Check sheet for the modelled part. Datum: model origin and axes. Units: mm. A direction names the side the tool comes from. Give positions to 0.01 mm unless a question says otherwise; leave off trailing zeros. Write each loop counter-clockwise with the first axis right and the second up, starting at its lowest first coordinate (ties: lowest second). Pieces come first, ordered by that corner, then holes. Notation, with made-up numbers: M 1.25,-13.75 L 42.25,-13.75 A27 ccw 42.25,5.25 Z; hole C 37.25,-22.5 d3. An arc over 180 degrees is marked long. Write item = value, one per line. Start each with the question number.
1) Go/stop test with a flat-tipped pin: pin 1 (12.5 mm diameter, centred on x = -1, z = 11.5, fed in from -Y). Record where the tip stops, or that it passes through.
2) Mould release check, pull along Y, two halves, no side actions. Record for faces 3 (the flat face through (-25.171, 7.087, 12.325)), 4 (the cylindrical face through (35.1, -3.2, 9.4)), 5 (the flat face through (25, -7, 12)): released by +Y, released by -Y, zero draft, split by the parting line, or undercut.
3) Cross-section at B-B, the plane y = -5. Give the number of separate pieces and of enclosed holes in the cut face, plus the area to 3 significant figures.
4) Scan lines: line 1 along Z through (x, y) = (37.75, -3.1); line 2 along X through (y, z) = (-7.75, 22.5); line 3 along Z through (x, y) = (38.5, -5). Record each from-to range of solid material in increasing order. Write a range as [from, to].
5) Access from +Z, -Z, +X, -X, +Y, -Y to the whole of each face (thin tool, end or side, straight path). Record for faces 1 (the flat face through (-1, 3, 0)), 2 (the flat face through (-25, -7, 12)).
6) Cross-section at D-D, the plane x = 30. Record the cut outline in (y, z).
7) Cross-section at A-A, the plane z = 4.5. Record the cut outline in (x, y).
8) Cross-section at C-C, the plane x = -28. Record the cut outline in (y, z), plus the area to 3 significant figures.
Autodesk Inventor part; units mm, degrees
ref_plane "YZ Plane" through (0, 0, 0) normal (1, 0, 0) x (0, 1, 0)
ref_plane "XZ Plane" through (0, 0, 0) normal (0, 1, 0) x (-1, 0, 0)
ref_plane "XY Plane" through (0, 0, 0) normal (0, 0, 1) x (1, 0, 0)
sketch "Skizze1" plane through (0, 0, 0) normal (0, 0, 1) x (1, 0, 0)
  line L0 (-63, 0) -> (63, 0)
  line L1 (0, -6) -> (0, 18.5)
  arc A0 (5.8901, 13.979) -> (-5.8901, 13.979) centre (0, -2.5) ccw
  line L2 (-5.8901, 13.979) -> (-45, 0)
  line L3 (5.8901, 13.979) -> (45, 0)
  line L4 (-45, 0) -> (45, 0)
  dimension "d2" = 35
  dimension "d3" = 15
  dimension "d4" = 45
extrude "Extrusion1" add sketch "Skizze1" along normal blind 25
sketch "Skizze4" plane through (-45, 0, 0) normal (0, -1, 0) x (1, 0, 0)
  line L0 (0, 25) -> (90, 25)
  line L1 (0, 0) -> (0, 25)
  line L2 (90, 25) -> (0, 25)
  line L3 (0, 25) -> (0, 0)
  line L4 (0, 0) -> (90, 0)
  line L5 (90, 0) -> (90, 25)
  point P0 (45, 0)
extrude "Extrusion4" add sketch "Skizze4" along normal blind 10
sketch "Skizze5" plane through (-45, -10, 0) normal (-1, 0, 0) x (0, 0, 1)
  line L0 (25, 0) -> (0, 0)
  line L1 (0, 10) -> (0, 0)
  point P0 (4.5, 5)
  point P1 (20.5, 5)
  dimension "d17" = 5
  dimension "d18" = 5
  dimension "d19" = 25
  dimension "d20" = 16
  dimension "d21" = 4.5
hole "Bohrung1" at (-45, -5, 4.5) at (-45, -5, 20.5) direction (1, 0, 0) diameter 6 end through all
sketch "Skizze6" plane through (-45, -10, 0) normal (-1, 0, 0) x (0, 0, 1)
  line L0 (0, 10) -> (25, 10)
  line L1 (0, 23.979) -> (0, 10)
  point P0 (12.5, 6.9)
  dimension "d29" = 3.1
  dimension "d30" = 12.5
hole "Bohrung2" at (-45, -3.1, 12.5) direction (1, 0, 0) diameter 6.2 end through all
sketch "Skizze7" plane through (0, 0, 0) normal (0, 0, -1) x (-1, 0, 0)
  line L0 (0, -15) -> (0, 20)
  line L1 (45, -10) -> (-45, -10)
  line L2 (-25, -10) -> (25, -10)
  line L3 (25, -10) -> (25, 1)
  line L4 (25, 1) -> (-25, 1)
  line L5 (-25, 1) -> (-25, -10)
  point P0 (0, 0)
  dimension "d38" = 50
  dimension "d39" = 11
extrude "Extrusion5" cut sketch "Skizze7" against normal blind 25
properties part number "Schieber"
Reply:
q1.pin_1 = 1
q2.face_3 = released by +Y
q2.face_4 = undercut
q2.face_5 = zero draft
q3.separate_pieces = 8
q3.enclosed_holes = 0
q3.area = 324 mm2
q4.line_1 = [0, 2.18], [6.82, 9.4], [15.6, 18.18], [22.82, 25]
q4.line_2 = [-45, -25], [25, 45]
q4.line_3 = [0, 1.5], [7.5, 10.05], [14.95, 17.5], [23.5, 25]
q5.face_1 = -Z, +X, -X, +Y, -Y
q5.face_2 = +Z, -Z, -Y
q6.outline = M -10,0 L 5.36,0 L 5.36,25 L -10,25 Z; hole C -5,4.5 d6; hole C -5,20.5 d6; hole C -3.1,12.5 d6.2
q7.outline = M -45,-10 L -25,-10 L -25,-8 L -45,-8 Z; M -45,-2 L -25,-2 L -25,1 L 25,1 L 25,-2 L 45,-2 L 45,0 L 5.89,13.98 A17.5 ccw -5.89,13.98 L -45,0 Z; M 25,-10 L 45,-10 L 45,-8 L 25,-8 Z
q8.outline = M -10,0 L 6.08,0 L 6.08,25 L -10,25 Z; hole C -5,4.5 d6; hole C -5,20.5 d6; hole C -3.1,12.5 d6.2
q8.area = 315 mm2
